Read the model definition and answer for the solid it produces. Units are mm, in the model's axes. Give positions to 0.01 mm unless a question says otherwise; leave off trailing zeros. Write each loop counter-clockwise with the first axis right and the second up, starting at its lowest first coordinate (ties: lowest second). Pieces come first, ordered by that corner, then holes. Notation, with made-up numbers: (75.5, 13.5) - (119.5, 13.5) arc R13 ccw to (119.5, 20.5) - close; hole circle Ø1 at (-36.75, 87.25). An arc over 180 degrees is marked (long way). Use CSV: the item, a comma, the result in double quotes. Start each with the question number.
from build123d import *

# Parameters (mm, degrees)
F0_W     = 30
F0_H     = 30
F1_DEPTH = 800
F2_DEPTH = 12
F0_H_2   = 1170
F3_DEPTH = 12


with BuildPart() as f1:
    # F0 (on Front) → F1 (new body)
    with BuildSketch(Plane.XZ):
        with Locations((-935, 935)):
            Rectangle(F0_W, F0_H)
    extrude(amount=F1_DEPTH)



with BuildPart() as f1b:
    # F0 (on Front) → F1, piece 2 (new body)
    with BuildSketch(Plane.XZ):
        with Locations((935, 935)):
            Rectangle(F0_W, F0_H)
    extrude(amount=F1_DEPTH)


with BuildPart() as f1c:
    # F0 (on Front) → F1, piece 3 (new body)
    with BuildSketch(Plane.XZ):
        with Locations((935, 265)):
            Rectangle(F0_W, F0_H)
    extrude(amount=F1_DEPTH)


with BuildPart() as f1d:
    # F0 (on Front) → F1, piece 4 (new body)
    with BuildSketch(Plane.XZ):
        with Locations((335, 265)):
            Rectangle(F0_W, F0_H)
    extrude(amount=F1_DEPTH)


with BuildPart() as f1e:
    # F0 (on Front) → F1, piece 5 (new body)
    with BuildSketch(Plane.XZ):
        with Locations((335, -935)):
            Rectangle(F0_W, F0_H)
    extrude(amount=F1_DEPTH)


with BuildPart() as f1f:
    # F0 (on Front) → F1, piece 6 (new body)
    with BuildSketch(Plane.XZ):
        with Locations((-935, -935)):
            Rectangle(F0_W, F0_H)
    extrude(amount=F1_DEPTH)


with BuildPart() as f1_1:
    add(f1.part)

    add(f1b.part)  # F2 merges F1b

    add(f1c.part)  # F2 merges F1c

    add(f1d.part)  # F2 merges F1d

    add(f1e.part)  # F2 merges F1e

    add(f1f.part)  # F2 merges F1f
    # F0 (on Front) → F2 (join)
    with BuildSketch(Plane.XZ):
        Polygon((-920, -920), (-920, -950), (320, -950), (320, -920), (320, 250), (320, 280), (350, 280), (350, 250), (920, 250), (920, 280), (950, 280), (950, 920), (920, 920), (920, 950), (-920, 950), (-920, 920), (-950, 920), (-950, -920), align=None)
    extrude(amount=F2_DEPTH)

    # F0 (on Front) → F3 (join)
    with BuildSketch(Plane.XZ):
        Polygon((-920, -920), (-920, -950), (320, -950), (320, -920), (320, 250), (320, 280), (350, 280), (350, 250), (920, 250), (920, 280), (950, 280), (950, 920), (920, 920), (920, 950), (-920, 950), (-920, 920), (-950, 920), (-950, -920), align=None)
        with Locations((335, -335)):
            Rectangle(F0_W, F0_H_2)
        with Locations((335, -935)):
            Rectangle(F0_W, F0_H)
        with Locations((335, 265)):
            Rectangle(F0_W, F0_H)
        with Locations((935, 265)):
            Rectangle(F0_W, F0_H)
        with Locations((-935, -935)):
            Rectangle(F0_W, F0_H)
        with Locations((935, 935)):
            Rectangle(F0_W, F0_H)
        with Locations((-935, 935)):
            Rectangle(F0_W, F0_H)
    extrude(amount=F3_DEPTH)


solid = f1_1.part
(1) The part is cut by section B-B on z = 740. Write down the section's boundary in (x, y).
(2) The part is cut by section A-A on y = -387.5. Write down the section's boundary in (x, z).
(3) The part is cut by section C-C on x = -561. Write down the section's boundary in (y, z).
(4) Given P1, Ø3, axis at x = -249.5, z = -415.5, coming from the -Y side; P2, Ø24, axis at x = 342, y = -209.5, coming from the +Z side; P3, Ø15, axis at x = 935, y = -301, coming from the -Z side, each flat-ended and moving along its own axis, determine where each tip first touches the part or whether it passes through.
(5) Consider probe 1 along Y at (x, z) = (-488.5, 41). Determine where the line is inside the solid, lowest interval first.
Reported:
1,outline,"(-950, -12) - (950, -12) - (950, 0) - (-950, 0) - close"
2,outline,"(-950, -950) - (-920, -950) - (-920, -920) - (-950, -920) - close; (-950, 920) - (-920, 920) - (-920, 950) - (-950, 950) - close; (320, -950) - (350, -950) - (350, -920) - (320, -920) - close; (320, 250) - (350, 250) - (350, 280) - (320, 280) - close; (920, 250) - (950, 250) - (950, 280) - (920, 280) - close; (920, 920) - (950, 920) - (950, 950) - (920, 950) - close"
3,outline,"(-12, -950) - (0, -950) - (0, 950) - (-12, 950) - close"
4,P1,"y = -12"
4,P2,"z = 280"
4,P3,"z = 250"
5,probe 1,"-12 to 0"
